```python
from build123d import *

# Parameters (mm, degrees)
F0_R     = 11.815332
F1_DEPTH = 35
F2_R     = 5
F4_DEPTH = 40


with BuildPart() as f1:
    # F0 (on Front) → F1 (new body)
    with BuildSketch(Plane.XZ):
        with BuildLine():
            Line((47.136076, 23.104757), (-63.083914, 23.104757))
            ThreePointArc((-63.083914, 23.104757), (-80.926867, -14.680376), (-40.412867, -4.447924))
            ThreePointArc((-40.412867, -4.447924), (-37.739192, 0.091286), (-33.111934, 2.609511))
            Line((-33.111934, 2.609511), (47.136076, 2.609511))
            Line((47.136076, 2.609511), (47.136076, 23.104757))
        make_face()
        with Locations((-63.085444, 0)):
            Circle(F0_R, mode=Mode.SUBTRACT)
    extrude(amount=F1_DEPTH)

    # F2
    f2_edges = [f1.edges().sort_by_distance(p)[0] for p in [
        (47.136076, -35, 12.857134),
        (47.136076, 0, 12.857134),
    ]]
    fillet(f2_edges, radius=F2_R)

    # F3 (on face) → F4 (cut)
    with BuildSketch(Plane(origin=(0, 0, 2.609511), x_dir=(1, 0, 0), z_dir=(0, 0, -1))):
        with BuildLine():
            Line((47.136076, 12.5), (47.136076, 22.5))
            Line((47.136076, 22.5), (3.855412, 22.5))
            ThreePointArc((3.855412, 22.5), (-1.144588, 17.5), (3.855412, 12.5))
            Line((3.855412, 12.5), (47.136076, 12.5))
        make_face()
    extrude(amount=-F4_DEPTH, mode=Mode.SUBTRACT)


solid = f1.part
```
The model under review builds one solid part; all positions refer to its coordinate system, in mm. A direction names the side the tool comes from. Give positions to 0.01 mm unless a question says otherwise; leave off trailing zeros. Write each loop counter-clockwise with the first axis right and the second up, starting at its lowest first coordinate (ties: lowest second). Pieces come first, ordered by that corner, then holes. Notation, with made-up numbers: M 6.5,-15.75 L 57.5,-15.75 A20 cw 57.5,-1.75 Z; hole C -37.5,75 d9. An arc over 180 degrees is marked long. Answer in a Markdown table with one row per item.
Item 1: For line 1 along Y through (x, z) = (32, 13.5); line 2 along Z through (x, y) = (-16, -11.5); line 3 along Z through (x, y) = (-57.5, -3.5), list the stretches that pass through material, from the lowest coordinate up.
Check sheet entries:
| item | result |
|---|---|
| line 1 | -35 to -22.5, -12.5 to 0 |
| line 2 | 2.61 to 23.1 |
| line 3 | -22.42 to -10.41, 10.41 to 23.1 |
Item 2: Add section D-D on z = 13. Give the boundary of the cut face in (x, y), plus the area to 3 significant figures.
Check sheet entries:
| item | result |
|---|---|
| outline | M -82.19,-35 L 42.14,-35 A5 ccw 47.14,-30 L 47.14,-22.5 L 3.86,-22.5 A5 cw 3.86,-12.5 L 47.14,-12.5 L 47.14,-5 A5 ccw 42.14,0 L -82.19,0 Z |
| area | 4,040 mm2 |
Item 3: Add section B-B on z = -7. Give the boundary of the cut face in (x, y).
Check sheet entries:
| item | result |
|---|---|
| outline | M -85.1,-35 L -72.6,-35 L -72.6,0 L -85.1,0 Z; M -53.57,-35 L -41.07,-35 L -41.07,0 L -53.57,0 Z |
Item 4: Draft analysis for pull direction Z (two halves, no side actions). For faces 1 (the face through (-7, -17, 23.105)), 2 (the face through (-23, -35, 11)), 3 (the face through (-51.8, -17.3, 3.5)), 4 (the face through (-37.79, -17.26, 0.04)), state which applies: +Z half, -Z half, draft (parallel to the pull), parting line (faces both ways), or undercut.
Check sheet entries:
| item | result |
|---|---|
| face 1 | +Z half |
| face 2 | draft |
| face 3 | undercut |
| face 4 | -Z half |
Item 5: Add section A-A on x = 5.5. Give the boundary of the cut face in (y, z).
Check sheet entries:
| item | result |
|---|---|
| outline | M -35,2.61 L -22.5,2.61 L -22.5,23.1 L -35,23.1 Z; M -12.5,2.61 L 0,2.61 L 0,23.1 L -12.5,23.1 Z |
Item 6: Add section C-C on y = -9. Give the boundary of the cut face in (x, z).
Check sheet entries:
| item | result |
|---|---|
| outline | M -63.08,23.1 A23.1 ccw long -40.41,-4.45 A9.87 cw -33.11,2.61 L 47.14,2.61 L 47.14,23.1 Z; hole C -63.09,0 d23.63 |
Item 7: Tool access review of faces 5 (the face through (-23, 0, 11)), 6 (the face through (25, -12.5, 13)), 7 (the face through (-2, -17, 2.61)): name each direction out of +Z, -Z, +X, -X, +Y, -Y from which nothing blocks a thin tool from reaching the whole face with its end or side.
Check sheet entries:
| item | result |
|---|---|
| face 5 | +Z, -Z, +X, -X, +Y |
| face 6 | +Z, -Z, +X |
| face 7 | -Z, +X, +Y, -Y |
Item 8: For P1, Ø12, axis at x = 6.5, y = -20.5, coming from the -Z side; P2, Ø4, axis at y = -28.5, z = 17.5, coming from the -X side, all flat-tipped, find the tip position at first contact; note any pin that passes through.
Check sheet entries:
| item | result |
|---|---|
| P1 | z = 2.61 |
| P2 | x = -80.22 |
